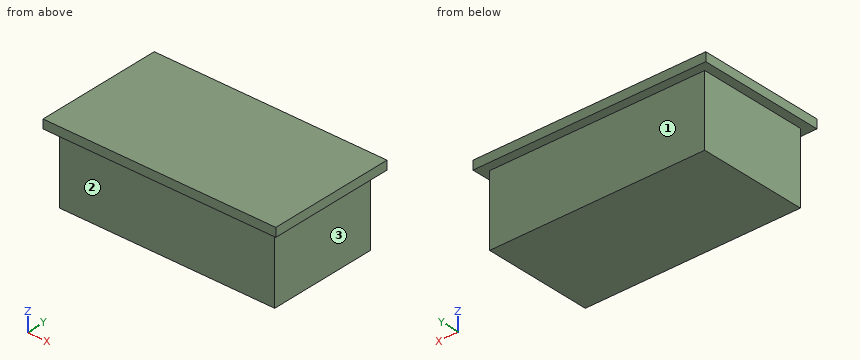
```python
from build123d import *

# Parameters (mm, degrees)
SKIZZE1_W                       = 79
SKIZZE1_H                       = 43
AUFSATZ_LINEAR_AUSTRAGEN1_DEPTH = 27
SKIZZE2_W                       = 79
SKIZZE2_H                       = 43
SKIZZE2_W_2                     = 73
SKIZZE2_H_2                     = 37
SCHNITT_LINEAR_AUSTRAGEN1_DEPTH = 24


with BuildPart() as part:
    # Skizze1 → Aufsatz-Linear austragen1 (new body)
    with BuildSketch(Plane.XY):
        Rectangle(SKIZZE1_W, SKIZZE1_H)
    extrude(amount=AUFSATZ_LINEAR_AUSTRAGEN1_DEPTH)

    # Skizze2 → Schnitt-Linear austragen1 (cut)
    with BuildSketch(Plane(origin=(0, 0, 0), x_dir=(-1, 0, 0), z_dir=(0, 0, -1))):
        Rectangle(SKIZZE2_W, SKIZZE2_H)
        Rectangle(SKIZZE2_W_2, SKIZZE2_H_2, mode=Mode.SUBTRACT)
    extrude(amount=-SCHNITT_LINEAR_AUSTRAGEN1_DEPTH, mode=Mode.SUBTRACT)


solid = part.part
```
Read the model definition and answer for the solid it produces. Units are mm, in the model's axes. Face numbers are marked on the shaded views. A direction names the side the tool comes from. Give positions to 0.01 mm unless a question says otherwise; leave off trailing zeros. Order: outer loops, then holes, each group sorted by start corner. A loop starts at its lowest first (then second) coordinate and runs counter-clockwise, first axis right, second up. Notation, with made-up numbers: (41.25, -18.5) -> (56.25, -18.5) arc R23 cw to (56.25, -6.5) -> close; hole circle Ø4 at (34.5, 35). An arc over 180 degrees is marked (long way). One line per item, written item: value. Start each with the question number.
(1) A tool of negligible diameter and unlimited length cuts with its end or side. For the marked faces 1, 2 and 3, from which of +Z, -Z, +X, -X, +Y, -Y can it reach the whole face along a straight path? Write none if from no direction.
(2) The part is cut by section C-C (z = 2). Determine the outline of the cut face in (x, y), and give its area (3 significant figures).
(3) The part is cut by section B-B (x = 20). Determine the outline of the cut face in (y, z).
(4) The part is cut by section A-A (y = 15). Determine the outline of the cut face in (x, z).
(5) Straight lines are drawn through the part: L1, parallel to Y at x = -20, z = 5.5; L2, parallel to X at y = 6, z = 12; L3, parallel to Z at x = 7.5, y = -19. For each, find the intervals that lie inside material, in ascending order.
(6) Flat-ended cylindrical pins translate along their axes: P1, Ø8, axis at x = -15.5, z = 3, coming from the +Y side; P2, Ø12, axis at y = 1.5, z = 17, coming from the -X side; P3, Ø12, axis at x = 26.5, z = 15.5, coming from the -Y side. Find the tip coordinate at first contact, or state that the pin passes through.
Taken from the geometry:
1. face 1: -Z, +X, -X, +Y
1. face 2: -Z, +X, -X, -Y
1. face 3: -Z, +X, +Y, -Y
2. outline: (-36.5, -18.5) -> (36.5, -18.5) -> (36.5, 18.5) -> (-36.5, 18.5) -> close
2. area: 2,700 mm^2
3. outline: (-21.5, 24) -> (-18.5, 24) -> (-18.5, 0) -> (18.5, 0) -> (18.5, 24) -> (21.5, 24) -> (21.5, 27) -> (-21.5, 27) -> close
4. outline: (-39.5, 24) -> (-36.5, 24) -> (-36.5, 0) -> (36.5, 0) -> (36.5, 24) -> (39.5, 24) -> (39.5, 27) -> (-39.5, 27) -> close
5. L1: -18.5 to 18.5
5. L2: -36.5 to 36.5
5. L3: 24 to 27
6. P1: y = 18.5
6. P2: x = -36.5
6. P3: y = -18.5
